Check sheet for the modelled part. Datum: model origin and axes. Units: mm. Face numbers are marked on the shaded views. A direction names the side the tool comes from. Give positions to 0.01 mm unless a question says otherwise; leave off trailing zeros. Loops run counter-clockwise (first coordinate to the right, second up) from the corner with the lowest first, then second, coordinate; pieces in that order, holes last. Notation, with made-up numbers: M 85.5,56 L 134.5,56 A29 ccw 134.5,79 Z; hole C 67,-38.5 d2. An arc over 180 degrees is marked long. One line per question, with ' | ' between items. Start each with the question number.
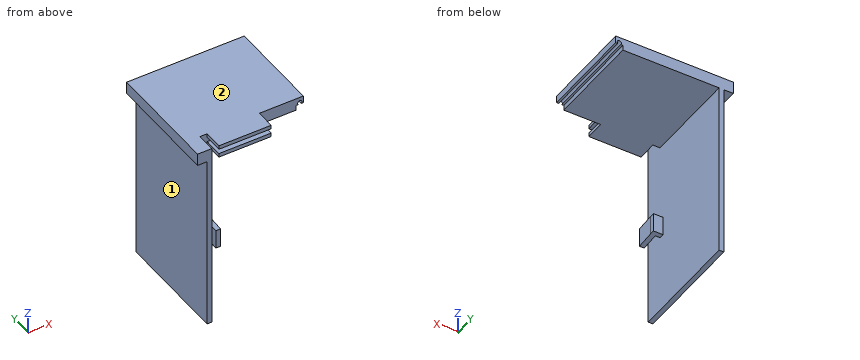
from build123d import *

# Parameters (mm, degrees)
BOSS_EXTRUDE1_DEPTH = 76.2
SKETCH9_W           = 6.35
SKETCH9_H           = 60.325
CUT_EXTRUDE1_DEPTH  = 65.7225
CUT_EXTRUDE2_DEPTH  = 12.7
LEFTCUT_DEPTH       = 76.2


# Read off the part's stored shape, not the designer's step: LeftCut
with BuildPart() as part:
    # Sketch8 → Boss-Extrude1 (new body)
    with BuildSketch(Plane(origin=(0, 0, 0), x_dir=(1, 0, 0), z_dir=(0, 1, 0))):
        Polygon((66.675, 8.255), (-66.675, 8.255), (-66.675, 61.2775), (-60.325, 61.2775), (-60.325, 73.9775), (-66.675, 73.9775), (-66.675, 127), (-69.85, 127), (-69.85, 8.255), (-76.2, 8.255), (-76.2, 0), (76.2, 0), (76.2, 8.255), (69.85, 8.255), (69.85, 127), (66.675, 127), (66.675, 73.9775), (60.325, 73.9775), (60.325, 61.2775), (66.675, 61.2775), align=None)
    extrude(amount=BOSS_EXTRUDE1_DEPTH)

    # Sketch9 → Cut-Extrude1 (cut)
    with BuildSketch(Plane(origin=(0, 0, -73.9775), x_dir=(-1, 0, 0), z_dir=(0, 0, -1))):
        Polygon((-66.675, 12.7), (-66.675, 0), (-64.008, 0), (-63.5, 12.7), align=None)
        Polygon((66.675, 12.7), (63.5, 12.7), (64.008, 0), (66.675, 0), align=None)
        with Locations((-63.5, 46.0375)):
            Rectangle(SKETCH9_W, SKETCH9_H)
        Polygon((-60.325, 0), (-60.325, 12.7), (-60.833, 0), align=None)
        Polygon((-60.198, 15.875), (-60.325, 15.875), (-60.325, 12.7), align=None)
        Polygon((60.833, 0), (60.325, 12.7), (60.325, 0), align=None)
        Polygon((60.325, 12.7), (60.325, 15.875), (60.198, 15.875), align=None)
        with Locations((63.5, 46.0375)):
            Rectangle(SKETCH9_W, SKETCH9_H)
    extrude(amount=-CUT_EXTRUDE1_DEPTH, mode=Mode.SUBTRACT)

    # Sketch10 → Cut-Extrude2 (cut)
    with BuildSketch(Plane.XZ):
        Polygon((26.9875, -5.715), (61.9125, -5.715), (61.9125, -8.255), (66.675, -8.255), (66.675, 0), (61.9125, 0), (61.9125, -2.54), (26.9875, -2.54), (26.9875, 0), (-26.9875, 0), (-26.9875, -2.54), (-61.9125, -2.54), (-61.9125, 0), (-66.675, 0), (-66.675, -8.255), (-61.9125, -8.255), (-61.9125, -5.715), (-26.9875, -5.715), (-26.9875, -8.255), (26.9875, -8.255), align=None)
    extrude(amount=-CUT_EXTRUDE2_DEPTH, mode=Mode.SUBTRACT)

    # LeftCut outline → LeftCut (cut)
    with BuildSketch(Plane(origin=(0, 0, 0), x_dir=(1, 0, 0), z_dir=(0, 1, 0))):
        with BuildLine():
            ThreePointArc((-0.98425, 4.801393432), (0, 2.413), (0.98425, 4.801393432))
            Line((0.98425, 4.801393432), (2.38125, 4.801393432))
            Line((2.38125, 4.801393432), (2.38125, 0))
            Line((2.38125, 0), (76.2, 0))
            Line((76.2, 0), (76.2, 8.255))
            Line((76.2, 8.255), (69.85, 8.255))
            Line((69.85, 8.255), (69.85, 127))
            Line((69.85, 127), (66.675, 127))
            Line((66.675, 127), (66.675, 73.9775))
            Line((66.675, 73.9775), (60.325, 73.9775))
            Line((60.325, 73.9775), (60.325, 61.2775))
            Line((60.325, 61.2775), (66.675, 61.2775))
            Line((66.675, 61.2775), (66.675, 8.255))
            Line((66.675, 8.255), (-2.38125, 8.255))
            Line((-2.38125, 8.255), (-2.38125, 4.801393432))
            Line((-2.38125, 4.801393432), (-0.98425, 4.801393432))
        make_face()
    extrude(amount=LEFTCUT_DEPTH, mode=Mode.SUBTRACT)


solid = part.part
Q1. Cross-section at A-A (y = 18). Record the cut outline in (x, z) (3 decimals).
Q2. Cross-section at C-C (z = -50). Record the cut outline in (x, y) (3 decimals), and give its area (3 significant figures).
Q3. Cross-section at B-B (x = -52.5). Record the cut outline in (y, z) (3 decimals).
Q4. Access from +Z, -Z, +X, -X, +Y, -Y to the whole of each face (thin tool, end or side, straight path). Record for the marked faces 1 and 2.
Q5. Material ranges on probe 1 along X at (y, z) = (56.5, -3.81); probe 2 along X at (y, z) = (5, -6.5) (1 decimal); probe 3 along Z at (x, y) = (-38, 12) (3 decimals), recorded low to high. Write a range as from..to.
Q6. Depth check by flat-ended pin: P1, Ø5, axis at y = 60, z = -69, coming from the -X side; P2, Ø1.9, axis at x = -65, z = -68, coming from the +Y side (3 decimals); P3, Ø4.5, axis at x = 0, z = -3.81, coming from the -Y side. Enter the tip coordinate at first touch or a pass-through.
Solved:
1) outline: M -76.2,-8.255 L -69.85,-8.255 L -69.85,-127 L -66.675,-127 L -66.675,-8.255 L -2.381,-8.255 L -2.381,-4.801 L -0.984,-4.801 A1.397 cw long 0.984,-4.801 L 2.381,-4.801 L 2.381,0 L -76.2,0 Z
2) outline: M -69.85,0 L -66.675,0 L -66.675,76.2 L -69.85,76.2 Z | area: 242 mm²
3) outline: M 0,-8.255 L 76.2,-8.255 L 76.2,0 L 0,0 L 0,-2.54 L 12.7,-2.54 L 12.7,-5.715 L 0,-5.715 Z
4) face 1: -Z, -X, +Y, -Y | face 2: +Z, +X, -X, +Y, -Y
5) probe 1: x = -76.2..-1.4, 1.4..2.38 | probe 2: x = -76.2..-66.7, -61.9..-27 | probe 3: z = -8.255..-5.715, -2.54..0
6) P1: stops at x = -69.85 | P2: stops at y = 15.875 | P3: stops at y = 12.7
